```python
from build123d import *

# Parameters (mm, degrees)
SKETCH1_W           = 45.72
SKETCH1_H           = 12.7
BOSS_EXTRUDE1_DEPTH = 9.652
CUT_EXTRUDE3_DEPTH  = 3.556
CUT_EXTRUDE5_DEPTH  = 25.496189826
SKETCH4_R           = 2
CUT_EXTRUDE6_DEPTH  = 28.875270474


with BuildPart() as part:
    # Sketch1 → Boss-Extrude1 (new body)
    with BuildSketch(Plane.XY):
        Rectangle(SKETCH1_W, SKETCH1_H)
    extrude(amount=BOSS_EXTRUDE1_DEPTH)

    # Sketch2 → Cut-Extrude3 (cut)
    with BuildSketch(Plane.XY.offset(9.652)):
        with BuildLine():
            Line((-9.144, -6.35), (9.144, -6.35))
            ThreePointArc((9.144, -6.35), (0, 2.794), (-9.144, -6.35))
        make_face()
    extrude(amount=-CUT_EXTRUDE3_DEPTH, mode=Mode.SUBTRACT)

    # Sketch3 → Cut-Extrude5 (cut, through all)
    with BuildSketch(Plane.XY.offset(6.096)):
        with BuildLine():
            Line((-6.096, -6.35), (6.096, -6.35))
            ThreePointArc((6.096, -6.35), (0, -0.254), (-6.096, -6.35))
        make_face()
    extrude(amount=-CUT_EXTRUDE5_DEPTH, mode=Mode.SUBTRACT)

    # Sketch4 → Cut-Extrude6 (cut, through all)
    with BuildSketch(Plane(origin=(0, 6.35, 0), x_dir=(1, 0, 0), z_dir=(0, 1, 0))):
        with Locations(Location((-18.034, -4.826, 0), (0, 0, 270))):
            Circle(SKETCH4_R)
        with Locations(Location((18.034, -4.826, 0), (0, 0, 90))):
            Circle(SKETCH4_R)
    extrude(amount=-CUT_EXTRUDE6_DEPTH, mode=Mode.SUBTRACT)


solid = part.part
```
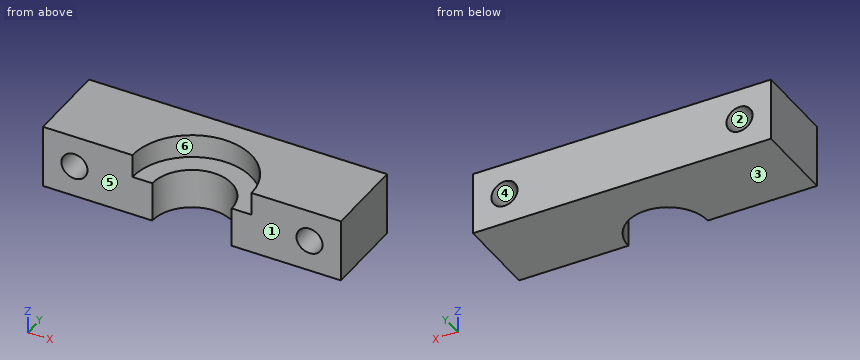
Verification items for the finished model (mm, model axes). Face numbers are marked on the shaded views. A direction names the side the tool comes from. Round coordinates to 2 decimals unless told otherwise and drop trailing zeros. Loops run counter-clockwise (first coordinate to the right, second up) from the corner with the lowest first, then second, coordinate; pieces in that order, holes last. Notation, with made-up numbers: (53, 70.5) -> (88, 70.5) arc R23 cw to (88, 103.5) -> close; hole circle Ø10 at (30, 70.5). An arc over 180 degrees is marked (long way). Answer as a JSON object with one key per item and string values.
Q1. Section check D-D (y = 4.5). Record the boundary of the cut face in (x, z), then the cut area to 3 significant figures.
Data:
{"outline": "(-22.86, 0) -> (22.86, 0) -> (22.86, 9.65) -> (-22.86, 9.65) -> close; hole circle Ø4 at (-18.03, 4.83); hole circle Ø4 at (18.03, 4.83)", "area": "416 mm2"}
Q2. Draft check along Z on the marked faces 1, 2, 3 and 4. Enter one of: pulls with the +Z half, pulls with the -Z half, needs draft (parallel to the pull), parting line crosses it, or undercut.
Data:
{"face 1": "needs draft", "face 2": "undercut", "face 3": "pulls with the -Z half", "face 4": "undercut"}
Q3. Section check A-A (y = -3.75). Record the boundary of the cut face in (x, z), then the cut area to 3 significant figures.
Data:
{"outline": "(-22.86, 0) -> (-5.51, 0) -> (-5.51, 6.1) -> (-8.77, 6.1) -> (-8.77, 9.65) -> (-22.86, 9.65) -> close; (5.51, 0) -> (22.86, 0) -> (22.86, 9.65) -> (8.77, 9.65) -> (8.77, 6.1) -> (5.51, 6.1) -> close; hole circle Ø4 at (-18.03, 4.83); hole circle Ø4 at (18.03, 4.83)", "area": "287 mm2"}
Q4. Section check B-B (z = 4). Record the boundary of the cut face in (x, y).
Data:
{"outline": "(-22.86, -6.35) -> (-19.86, -6.35) -> (-19.86, 6.35) -> (-22.86, 6.35) -> close; (-16.21, -6.35) -> (-6.1, -6.35) arc R6.1 cw to (6.1, -6.35) -> (16.21, -6.35) -> (16.21, 6.35) -> (-16.21, 6.35) -> close; (19.86, -6.35) -> (22.86, -6.35) -> (22.86, 6.35) -> (19.86, 6.35) -> close"}
Q5. Access from +Z, -Z, +X, -X, +Y, -Y to the whole of each face (thin tool, end or side, straight path). Record for the marked faces 5 and 6.
Data:
{"face 5": "+Z, -Z, +X, -X, -Y", "face 6": "+Z, -Y"}
Q6. Go/stop test with flat-tipped pins: P1, Ø4.5, axis at x = -18.034, z = 4.826, coming from the -Y side; P2, Ø2.5, axis at x = -4.5, y = 0, coming from the +Z side. Record where each tip stops, or that it passes through.
Data:
{"P1": "stops at y = -6.35", "P2": "stops at z = 6.1"}
Q7. Section check C-C (x = 0). Record the boundary of the cut face in (y, z), then the cut area to 3 significant figures.
Data:
{"outline": "(-0.25, 0) -> (6.35, 0) -> (6.35, 9.65) -> (2.79, 9.65) -> (2.79, 6.1) -> (-0.25, 6.1) -> close", "area": "52.9 mm2"}
Q8. Scan lines: line 1 (X direction, y = 4, z = 4.75); line 2 (Z direction, x = 18, y = 0.25); line 3 (X direction, y = 0, z = 4.5). Record each from-to range of solid material in increasing order. Write a range as from..to.
Data:
{"line 1": "x = -22.86..-20.03, -16.04..16.04, 20.03..22.86", "line 2": "z = 0..2.83, 6.83..9.65", "line 3": "x = -22.86..-20.01, -16.06..16.06, 20.01..22.86"}
